Check sheet for the modelled part. Datum: model origin and axes. Units: mm. Face numbers are marked on the shaded views. A direction names the side the tool comes from. Round coordinates to 2 decimals unless told otherwise and drop trailing zeros. Write each loop counter-clockwise with the first axis right and the second up, starting at its lowest first coordinate (ties: lowest second). Pieces come first, ordered by that corner, then holes. Notation, with made-up numbers: M -7.75,-7 L 13.25,-7 A19 cw 13.25,23 Z; hole C -4,61.25 d6. An arc over 180 degrees is marked long. Put each result on its own line as item: value.
```python
from build123d import *
from build123d.topology import SkipClean

# Parameters (mm, degrees)
SKETCH5_W            = 40
SKETCH5_H            = 15
BOSS_EXTRUDE2_DEPTH  = 17
SKETCH6_R            = 13
CUT_EXTRUDE4_DEPTH   = 10
SKETCH7_R            = 2.5
CUT_EXTRUDE5_DEPTH   = 4.5
CHAMFER8_SIZE        = 10
BOSS_EXTRUDE3_START  = -6.5
BOSS_EXTRUDE3_DEPTH  = 6.5
SKETCH8_R            = 4.8
CUT_EXTRUDE8_DEPTH   = 3
SKETCH9_W            = 2.5
SKETCH9_H            = 2
CUT_EXTRUDE7_DEPTH   = 52
SKETCH11_R           = 5
CUT_EXTRUDE9_DEPTH   = 45
SKETCH12_R           = 9
SKETCH12_R_2         = 5
CUT_EXTRUDE11_DEPTH  = 1.2
CUT_EXTRUDE12_DEPTH  = 53.810983706
BOSS_EXTRUDE4_START  = 1.3
BOSS_EXTRUDE4_DEPTH  = 1.3
BOSS_EXTRUDE8_START  = -33.4
BOSS_EXTRUDE8_DEPTH  = 1.3
BOSS_EXTRUDE9_DEPTH  = 1.5
BOSS_EXTRUDE10_START = -34.5
BOSS_EXTRUDE10_DEPTH = 1.5


# Read off the part's stored shape, not the designer's step: Boss-Extrude3
with BuildPart() as part:
    # Sketch5 → Boss-Extrude2 (new body)
    with BuildSketch(Plane.XY):
        with Locations((-20, 7.5)):
            Rectangle(SKETCH5_W, SKETCH5_H)
    boss_extrude2 = extrude(amount=BOSS_EXTRUDE2_DEPTH)

    # Sketch6 → Cut-Extrude4 (cut)
    with BuildSketch(Plane(origin=(0, 0, 0), x_dir=(-1, 0, 0), z_dir=(0, 0, -1))):
        with Locations((20, 15)):
            Circle(SKETCH6_R)
    cut_extrude4 = extrude(amount=-CUT_EXTRUDE4_DEPTH, mode=Mode.SUBTRACT)

    # Sketch7 → Cut-Extrude5 (cut)
    with BuildSketch(Plane.XY.offset(17)):
        with Locations((-20, 15)):
            Circle(SKETCH7_R)
    cut_extrude5 = extrude(amount=-CUT_EXTRUDE5_DEPTH, mode=Mode.SUBTRACT)

    # Mirror5: Boss-Extrude2, Cut-Extrude4, Cut-Extrude5 across plane
    with SkipClean():  # the faces are left unmerged after this step: merging them gives an invalid solid
        add(boss_extrude2.mirror(Plane.XY))
        add(cut_extrude4.mirror(Plane.XY), mode=Mode.SUBTRACT)
        add(cut_extrude5.mirror(Plane.XY), mode=Mode.SUBTRACT)
    add(part.part.scale(1), mode=Mode.REPLACE)  # the faces are merged on a copy

    # Chamfer8
    # the kernel refuses this chamfer: 10 mm, written as the material it takes off along each edge
    with BuildSketch(Plane(origin=(-40, 15, -42.71682988), x_dir=(0.9996219169112968, 0.027495876610586317, 0), z_dir=(0, 0, 1)), Plane(origin=(0, 15, 42.71682988), x_dir=(-0.9996219169112968, 0.027495876610586317, 0), z_dir=(0, 0, -1))) as chamfer8_piece_1:
        Polygon((CHAMFER8_SIZE * 0.999621916911, -CHAMFER8_SIZE * 0.0274958766106), (-CHAMFER8_SIZE * 0.0274958766106, -CHAMFER8_SIZE * 0.999621916911), (0, 0), align=None)
    extrude(amount=85.433659759, mode=Mode.SUBTRACT)

    # Boss-Extrude3 outline → Boss-Extrude3 (add)
    with BuildSketch(Plane.XY.offset(-10).offset(BOSS_EXTRUDE3_START)):
        with BuildLine():
            Line((-10, 30), (-30, 30))
            Line((-30, 30), (-30, 15))
            Line((-30, 15), (-22.5, 15))
            ThreePointArc((-22.5, 15), (-20, 12.5), (-17.5, 15))
            Line((-17.5, 15), (-10, 15))
            Line((-10, 15), (-10, 30))
        make_face()
    boss_extrude3 = extrude(amount=BOSS_EXTRUDE3_DEPTH)

    # Mirror6: Boss-Extrude3 across plane
    add(boss_extrude3.mirror(Plane(origin=(0, 0, 0), x_dir=(1, 0, 0), z_dir=(0, 0, -1))))

    # Sketch8 → Cut-Extrude8 (cut)
    with BuildSketch(Plane.XZ):
        with Locations(Location((-33, 11.5, 0), (0, 0, 270))):
            Circle(SKETCH8_R)
        with Locations(Location((-7, 11.5, 0), (0, 0, 90))):
            Circle(SKETCH8_R)
        with Locations(Location((-7, -11.5, 0), (0, 0, 270))):
            Circle(SKETCH8_R)
        with Locations(Location((-33, -11.5, 0), (0, 0, 90))):
            Circle(SKETCH8_R)
    extrude(amount=-CUT_EXTRUDE8_DEPTH, mode=Mode.SUBTRACT)

    # Sketch9 → Cut-Extrude7 (cut)
    with BuildSketch(Plane.XZ):
        with Locations((-12.75, 16)):
            Rectangle(SKETCH9_W, SKETCH9_H)
        with Locations((-27.25, 16)):
            Rectangle(SKETCH9_W, SKETCH9_H)
        with Locations((-12.75, -16)):
            Rectangle(SKETCH9_W, SKETCH9_H)
        with Locations((-27.25, -16)):
            Rectangle(SKETCH9_W, SKETCH9_H)
    extrude(amount=-CUT_EXTRUDE7_DEPTH, mode=Mode.SUBTRACT)

    # Sketch11 → Cut-Extrude9 (cut, symmetric)
    with BuildSketch(Plane(origin=(0, 0, 10), x_dir=(-1, 0, 0), z_dir=(0, 0, -1))):
        with Locations((20, 15)):
            Circle(SKETCH11_R)
    extrude(amount=CUT_EXTRUDE9_DEPTH, both=True, mode=Mode.SUBTRACT)

    # Sketch12 → Cut-Extrude11 (cut)
    with BuildSketch(Plane(origin=(0, 0, 10), x_dir=(-1, 0, 0), z_dir=(0, 0, -1))):
        with Locations((20, 15)):
            Circle(SKETCH12_R)
        with Locations((20, 15)):
            Circle(SKETCH12_R_2, mode=Mode.SUBTRACT)
    cut_extrude11 = extrude(amount=-CUT_EXTRUDE11_DEPTH, mode=Mode.SUBTRACT)

    # Mirror7: Cut-Extrude11 across plane
    add(cut_extrude11.mirror(Plane(origin=(0, 0, 0), x_dir=(1, 0, 0), z_dir=(0, 0, -1))), mode=Mode.SUBTRACT)

    # Sketch13 → Cut-Extrude12 (cut, through all)
    with BuildSketch(Plane.XZ):
        Polygon((-26, 15), (-28.5, 15), (-28.5, 17), (-40, 17), (-40, -17), (-28.5, -17), (-28.5, -15), (-26, -15), (-26, -17), (-14, -17), (-14, -15), (-11.5, -15), (-11.5, -17), (0, -17), (0, 17), (-11.5, 17), (-11.5, 15), (-14, 15), (-14, 17), (-26, 17), align=None)
        Polygon((-25.7, 14.7), (-28.8, 14.7), (-28.8, 16.7), (-39.7, 16.7), (-39.7, -16.7), (-28.8, -16.7), (-28.8, -14.7), (-25.7, -14.7), (-25.7, -16.7), (-14.3, -16.7), (-14.3, -14.7), (-11.2, -14.7), (-11.2, -16.7), (-0.3, -16.7), (-0.3, 16.7), (-11.2, 16.7), (-11.2, 14.7), (-14.3, 14.7), (-14.3, 16.7), (-25.7, 16.7), align=None, mode=Mode.SUBTRACT)
    extrude(amount=-CUT_EXTRUDE12_DEPTH, mode=Mode.SUBTRACT)

    # Sketch14 → Boss-Extrude4 (add)
    with SkipClean():  # the faces are left unmerged after this step: merging them gives an invalid solid
        with BuildSketch(Plane(origin=(0, 0, -16.7), x_dir=(-1, 0, 0), z_dir=(0, 0, -1)).offset(BOSS_EXTRUDE4_START)):
            with BuildLine():
                Line((15, 15), (14.3, 15))
                Line((14.3, 15), (14.3, 0))
                Line((14.3, 0), (25.7, 0))
                Line((25.7, 0), (25.7, 15))
                Line((25.7, 15), (25, 15))
                ThreePointArc((25, 15), (20, 10), (15, 15))
            make_face()
        extrude(amount=-BOSS_EXTRUDE4_DEPTH)
    add(part.part.scale(1), mode=Mode.REPLACE)  # the faces are merged on a copy

    # Sketch14<3> → Boss-Extrude8 (add)
    with BuildSketch(Plane(origin=(0, 0, -16.7), x_dir=(-1, 0, 0), z_dir=(0, 0, -1)).offset(BOSS_EXTRUDE8_START)):
        with BuildLine():
            Line((15, 15), (14.3, 15))
            Line((14.3, 15), (14.3, 0))
            Line((14.3, 0), (25.7, 0))
            Line((25.7, 0), (25.7, 15))
            Line((25.7, 15), (25, 15))
            ThreePointArc((25, 15), (20, 10), (15, 15))
        make_face()
    extrude(amount=-BOSS_EXTRUDE8_DEPTH)

    # Sketch16 → Boss-Extrude9 (add)
    with BuildSketch(Plane.XY.offset(16.5)):
        with BuildLine():
            Line((-25.7, 30), (-25.7, 15))
            Line((-25.7, 15), (-25, 15))
            ThreePointArc((-25, 15), (-20, 20), (-15, 15))
            Line((-15, 15), (-14.3, 15))
            Line((-14.3, 15), (-14.3, 30))
            Line((-14.3, 30), (-25.7, 30))
        make_face()
    extrude(amount=BOSS_EXTRUDE9_DEPTH)

    # Sketch16<2> → Boss-Extrude10 (add)
    with SkipClean():  # the faces are left unmerged after this step: merging them gives an invalid solid
        with BuildSketch(Plane.XY.offset(16.5).offset(BOSS_EXTRUDE10_START)):
            with BuildLine():
                Line((-25.7, 30), (-25.7, 15))
                Line((-25.7, 15), (-25, 15))
                ThreePointArc((-25, 15), (-20, 20), (-15, 15))
                Line((-15, 15), (-14.3, 15))
                Line((-14.3, 15), (-14.3, 30))
                Line((-14.3, 30), (-25.7, 30))
            make_face()
        extrude(amount=BOSS_EXTRUDE10_DEPTH)
    add(part.part.scale(1), mode=Mode.REPLACE)  # the faces are merged on a copy


solid = part.part
```
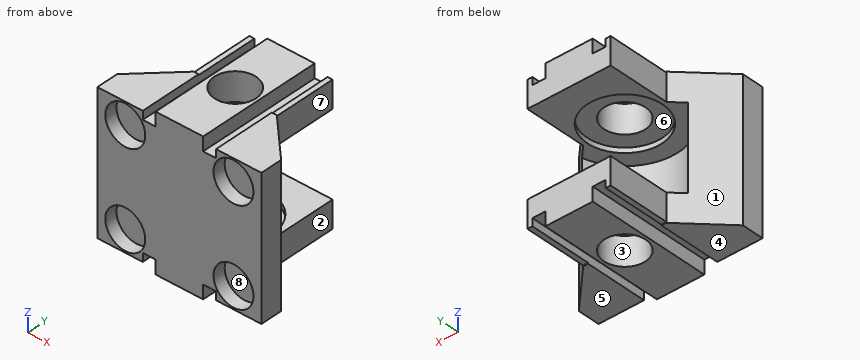
1. Access from +Z, -Z, +X, -X, +Y, -Y to the whole of each face (thin tool, end or side, straight path). Record for the marked faces 5, 6, 7 and 8.
Computed values:
face 5: -Z, +X, +Y, -Y
face 6: none
face 7: +Z, -Z, +X, +Y
face 8: -Y
2. Depth check by flat-ended pin: pin 1 Ø2 at (y, z) = (19.5, 16) entering from -X; pin 2 Ø6 at (y, z) = (9, -5) entering from -X; pin 3 Ø6 at (y, z) = (6, 2.5) entering from -X; pin 4 Ø4 at (x, y) = (-31.5, 26) entering from +Z. Enter the tip coordinate at first touch or a pass-through.
Computed values:
pin 1: stops at x = -30
pin 2: stops at x = -39
pin 3: stops at x = -39.7
pin 4: stops at z = 16.5
3. Cross-section at B-B (y = 28.25). Enter the section's corners in (x, z).
Computed values:
outline: M -30,-16.5 L -28.8,-16.5 L -28.8,-14.7 L -25.7,-14.7 L -25.7,-18 L -14.3,-18 L -14.3,-14.7 L -11.2,-14.7 L -11.2,-16.5 L -10,-16.5 L -10,-10 L -30,-10 Z; M -30,10 L -10,10 L -10,16.5 L -11.2,16.5 L -11.2,14.7 L -14.3,14.7 L -14.3,18 L -25.7,18 L -25.7,14.7 L -28.8,14.7 L -28.8,16.5 L -30,16.5 Z
4. Cross-section at D-D (x = -30.5). Enter the section's corners in (y, z).
Computed values:
outline: M 0,-16.7 L 14.5,-16.7 L 14.5,-10 L 7.34,-10 L 7.34,10 L 14.5,10 L 14.5,16.7 L 0,16.7 L 0,15.6 L 3,15.6 L 3,7.4 L 0,7.4 L 0,-7.4 L 3,-7.4 L 3,-15.6 L 0,-15.6 Z
5. Cross-section at C-C (z = 2). Enter the section's corners in (x, y), then the cut area to 3 significant figures.
Computed values:
outline: M -39.7,0 L -0.3,0 L -0.3,5.3 L -7.29,12.29 A13 cw -32.71,12.29 L -39.7,5.3 Z
area: 240 mm2
6. Cross-section at A-A (x = -20). Enter the section's corners in (y, z), then the cut area to 3 significant figures.
Computed values:
outline: M 0,-18 L 10,-18 L 10,-11.2 L 6,-11.2 L 6,-10 L 2,-10 L 2,10 L 6,10 L 6,11.2 L 10,11.2 L 10,18 L 0,18 Z; M 20,-18 L 30,-18 L 30,-10 L 24,-10 L 24,-11.2 L 20,-11.2 Z; M 20,11.2 L 24,11.2 L 24,10 L 30,10 L 30,18 L 20,18 Z
area: 341 mm2
7. Scan lines: probe 1 along X at (y, z) = (1.7, 11.5); probe 2 along Y at (x, z) = (-20, 10.8); probe 3 along Z at (x, y) = (-9, 11.5). Record each from-to range of solid material in increasing order.
Computed values:
probe 1: x = -39.7 to -37.8, -28.2 to -11.8, -2.2 to -0.3
probe 2: y = 0 to 6, 24 to 30
probe 3: z = -16.7 to -10, 10 to 16.7
8. Release check for a two-part mould opening along X. For the marked faces 1, 2, 3 and 4 record: +X half, -X half, draft (parallel to the pull), parting line (faces both ways), or undercut.
Computed values:
face 1: -X half
face 2: +X half
face 3: undercut
face 4: draft
